Input: part model. Units: mm. Frame: model coordinates. A direction names the side the tool comes from. Coordinates: 2 decimals unless noted, no trailing zeros. Loops run counter-clockwise (first coordinate to the right, second up) from the corner with the lowest first, then second, coordinate; pieces in that order, holes last.
(1) Contact query for flat-ended pins moving along their axis: P1, Ø0.8, axis at x = 0, y = 0, coming from the +Z side; P2, Ø2, axis at y = 1, z = -6.5, coming from the +X side; P3, Ø2, axis at y = -1.5, z = -5.5, coming from the -X side. Output: stop coordinate, or through.
(2) Section A-A, the plane z = 2. Return loops of the section in (x, y), then the cut area to 3 significant figures.
(3) Section B-B, the plane y = 0. Return loops of the section in (x, z).
(4) Mould query, pull axis Y, two halves, no side actions, for faces 1 (the face through (0, 0, -8)), 2 (the face through (1.5, 0.07, -3.94)), 3 (the face through (-0.63, -1.08, 2.26)). Classes: released by +Y, released by -Y, zero draft, split by the parting line, or undercut.
(5) Section C-C, the plane x = 0.15. Return loops of the section in (y, z), then the cut area to 3 significant figures.
(6) Line query: L1, parallel to X at y = 0.1, z = 2.5; L2, parallel to Z at x = -1.5, y = -1.3; L3, parallel to Z at x = -1.1, y = 0.2. Output: solid intervals per line, ascending.
(7) Section D-D, the plane z = -3. Return loops of the section in (x, y), then the cut area to 3 significant figures.
(8) Set-up query: faces 4 (the face through (-1.25, 0, 2)), 5 (the face through (0.6, 1.3, 3)), 6 (the face through (1.2, -1.2, 0)). Return all of +Z, -Z, +X, -X, +Y, -Y with unobstructed straight access to the full face (end or side cutting, diameter ignored); none if empty.
```python
from build123d import *

# Parameters (mm, degrees)
SKETCH_1_R          = 2.75
EXTRUDE_1_DEPTH     = 3
CUT_EXTRUDE_1_DEPTH = 1.5
SKETCH_3_R          = 1.5
EXTRUDE_2_DEPTH     = 8


with BuildPart() as part:
    # 草图1 → 凸台-拉伸1 (new body)
    with BuildSketch(Plane.XY):
        Circle(SKETCH_1_R)
    extrude(amount=EXTRUDE_1_DEPTH)

    # 草图2 → 切除-拉伸1 (cut)
    with BuildSketch(Plane.XY.offset(3)):
        Polygon((0, -1.443375673), (1.25, -0.721687836), (1.25, 0.721687836), (0, 1.443375673), (-1.25, 0.721687836), (-1.25, -0.721687836), align=None)
    extrude(amount=-CUT_EXTRUDE_1_DEPTH, mode=Mode.SUBTRACT)

    # 草图3 → 凸台-拉伸2 (add)
    with BuildSketch(Plane(origin=(0, 0, 0), x_dir=(-1, 0, 0), z_dir=(0, 0, -1))):
        Circle(SKETCH_3_R)
    extrude(amount=EXTRUDE_2_DEPTH)


solid = part.part
```
Report:
1. P1: stops at z = 1.5
1. P2: stops at x = 1.5
1. P3: stops at x = -1.41
2. outline: circle Ø5.5 at (0, 0); hole (-1.25, -0.72) - (0, -1.44) - (1.25, -0.72) - (1.25, 0.72) - (0, 1.44) - (-1.25, 0.72) - close
2. area: 18.3 mm2
3. outline: (-2.75, 0) - (-1.5, 0) - (-1.5, -8) - (1.5, -8) - (1.5, 0) - (2.75, 0) - (2.75, 3) - (1.25, 3) - (1.25, 1.5) - (-1.25, 1.5) - (-1.25, 3) - (-2.75, 3) - close
4. face 1: zero draft
4. face 2: split by the parting line
4. face 3: undercut
5. outline: (-2.75, 0) - (-1.49, 0) - (-1.49, -8) - (1.49, -8) - (1.49, 0) - (2.75, 0) - (2.75, 3) - (1.36, 3) - (1.36, 1.5) - (-1.36, 1.5) - (-1.36, 3) - (-2.75, 3) - close
5. area: 36.3 mm2
6. L1: x = -2.75 to -1.25, 1.25 to 2.75
6. L2: z = 0 to 3
6. L3: z = -8 to 1.5
7. outline: circle Ø3 at (0, 0)
7. area: 7.07 mm2
8. face 4: +Z
8. face 5: +Z, +X, -X, +Y, -Y
8. face 6: -Z
